Input: part model. Units: mm. Frame: model coordinates. A direction names the side the tool comes from. Round coordinates to 2 decimals unless told otherwise and drop trailing zeros. Loops run counter-clockwise (first coordinate to the right, second up) from the corner with the lowest first, then second, coordinate; pieces in that order, holes last.
1) Section B-B, the plane z = 2. Return loops of the section in (x, y) (3 decimals).
2) Ray query, line 1 along Z through (x, y) = (2.4, -0.8); line 2 along Z through (x, y) = (2.1, 0.55); line 3 along X through (y, z) = (0, 2.5) (3 decimals). Return the intervals inside material, ascending.
3) First-contact query: pin 1 (3 mm diameter, centred on x = -2, y = -1, fed in from -Z); pin 2 (1 mm diameter, centred on y = 1, z = 4.5, fed in from -X); pin 3 (3 mm diameter, centred on x = -2, y = -0.5, fed in from +Z); pin 4 (1 mm diameter, centred on y = 0, z = 3, fed in from +X) (3 decimals). Flat tips, straight axial feed; report the tip coordinate or a pass-through.
4) Section A-A, the plane y = 2.25. Return loops of the section in (x, z).
5) Access query for faces 1 (the face through (0, 0, 0)), 2 (the face through (-0.305, 2.325, 2.566)). Directions: +Z, -Z, +X, -X, +Y, -Y. A direction counts if a zero-diameter tool reaches every point of the face in a straight line with its end or side. Return the directions, or none.
from build123d import *

# Parameters (mm, degrees)
SKETCH_R     = 2.75
PAD_DEPTH    = 0.2
SKETCH002_R  = 2.345
PAD001_DEPTH = 5


with BuildPart() as part:
    # Sketch → Pad (new body)
    with BuildSketch(Plane.XY):
        Circle(SKETCH_R)
    extrude(amount=PAD_DEPTH)

    # Sketch002 → Pad001 (join)
    with BuildSketch(Plane.XY):
        Circle(SKETCH002_R)
    extrude(amount=PAD001_DEPTH)

    # Sketch003 → Revolution (revolve)
    with BuildSketch(Plane.YZ):
        with BuildLine():
            Line((0, 4.85), (0, 6.15))
            ThreePointArc((2.133073, 4.85), (1.249, 5.79939), (0, 6.15))
            Line((0, 4.85), (2.133073, 4.85))
        make_face()
    revolve(axis=Axis((0, 0, 0), (0, 0, 1)))


solid = part.part
Final values:
1. outline: circle Ø4.69 at (0, 0)
2. line 1: z = 0 to 0.2
2. line 2: z = 0 to 5
2. line 3: x = -2.345 to 2.345
3. pin 1: stops at z = 0
3. pin 2: stops at x = -2.29
3. pin 3: stops at z = 6.08
3. pin 4: stops at x = 2.345
4. outline: (-1.58, 0) - (1.58, 0) - (1.58, 0.2) - (0.66, 0.2) - (0.66, 5) - (-0.66, 5) - (-0.66, 0.2) - (-1.58, 0.2) - close
5. face 1: -Z, +X, -X, +Y, -Y
5. face 2: +Z
